CAD build for the part. Positions are in the model's coordinates, mm. Round coordinates to 2 decimals unless told otherwise and drop trailing zeros. Loops run counter-clockwise (first coordinate to the right, second up) from the corner with the lowest first, then second, coordinate; pieces in that order, holes last. Notation, with made-up numbers: (1.25, 47) - (9.25, 47) arc R28 ccw to (9.25, 67) - close; hole circle Ø10 at (50, 64). An arc over 180 degrees is marked (long way). Use one line per item in the form item = value.
from build123d import *

# Parameters (mm, degrees)
F0_R     = 1.5
F1_DEPTH = 1.5


with BuildPart() as f1:
    # F0 (on Top) → F1 (new body)
    with BuildSketch(Plane.XY):
        with BuildLine():
            ThreePointArc((-0.1201086231, 2.7473758241), (1.2696708079, 2.4393515613), (2.3192429637, 1.4777050029))
            Line((2.3192429637, 1.4777050029), (1.4660895902, 2.8167205482))
            Line((1.4660895902, 2.8167205482), (-0.1201086231, 2.7473758241))
        make_face()
        with BuildLine():
            Line((1.706306755, -2.6780311034), (2.4393515428, -1.2696708434))
            ThreePointArc((2.4393515428, -1.2696708434), (1.477704987, -2.3192429738), (0.1201085757, -2.7473758261))
            Line((0.1201085757, -2.7473758261), (1.706306755, -2.6780311034))
        make_face()
        with BuildLine():
            ThreePointArc((-2.4393515589, 1.2696708124), (-1.4777050217, 2.3192429516), (-0.1201086231, 2.7473758241))
            Line((-0.1201086231, 2.7473758241), (-1.706306755, 2.6780311034))
            Line((-1.706306755, 2.6780311034), (-2.4393515589, 1.2696708124))
        make_face()
        with BuildLine():
            ThreePointArc((2.3192429637, 1.4777050029), (2.6401153526, 0.7696043951), (2.75, 0))
            ThreePointArc((2.75, 0), (2.671209159, -0.6535607307), (2.4393515428, -1.2696708434))
            Line((2.4393515428, -1.2696708434), (3.1723963452, 0.1386894448))
            Line((3.1723963452, 0.1386894448), (2.3192429637, 1.4777050029))
        make_face()
        with BuildLine():
            Line((-1.4660895902, -2.8167205482), (0.1201085757, -2.7473758261))
            ThreePointArc((0.1201085757, -2.7473758261), (-1.2696708891, -2.439351519), (-2.3192430366, -1.4777048885))
            Line((-2.3192430366, -1.4777048885), (-1.4660895902, -2.8167205482))
        make_face()
        with BuildLine():
            ThreePointArc((-2.3192430366, -1.4777048885), (-2.7473758282, -0.1201085279), (-2.4393515589, 1.2696708124))
            Line((-2.4393515589, 1.2696708124), (-3.1723963452, -0.1386894448))
            Line((-3.1723963452, -0.1386894448), (-2.3192430366, -1.4777048885))
        make_face()
        with BuildLine():
            ThreePointArc((2.4393515428, -1.2696708434), (2.671209159, -0.6535607307), (2.75, 0))
            ThreePointArc((2.75, 0), (2.6401153526, 0.7696043951), (2.3192429637, 1.4777050029))
            ThreePointArc((2.3192429637, 1.4777050029), (1.2696708079, 2.4393515613), (-0.1201086231, 2.7473758241))
            ThreePointArc((-0.1201086231, 2.7473758241), (-1.4777050217, 2.3192429516), (-2.4393515589, 1.2696708124))
            ThreePointArc((-2.4393515589, 1.2696708124), (-2.7473758282, -0.1201085279), (-2.3192430366, -1.4777048885))
            ThreePointArc((-2.3192430366, -1.4777048885), (-1.2696708891, -2.439351519), (0.1201085757, -2.7473758261))
            ThreePointArc((0.1201085757, -2.7473758261), (1.477704987, -2.3192429738), (2.4393515428, -1.2696708434))
        make_face()
        Circle(F0_R, mode=Mode.SUBTRACT)
    extrude(amount=F1_DEPTH)


solid = f1.part
1) Slice it at B-B (y = 0.5). Write the cut outline in (x, z).
Report:
outline = (-2.84, 0) - (-1.41, 0) - (-1.41, 1.5) - (-2.84, 1.5) - close; (1.41, 0) - (2.94, 0) - (2.94, 1.5) - (1.41, 1.5) - close
2) Drill centre lines: probe 1 along X at (y, z) = (1.3, 0.1); probe 2 along X at (y, z) = (0.4, 0.45); probe 3 along Y at (x, z) = (0, 0.6). Where is each one in solid material? Low to high.
Report:
probe_1 = -2.42 to -0.75, 0.75 to 2.43
probe_2 = -2.89 to -1.45, 1.45 to 3.01
probe_3 = -2.75 to -1.5, 1.5 to 2.75
3) Slice it at D-D (x = 2). Write the cut outline in (y, z), plus the area to 3 significant figures.
Report:
outline = (-2.11, 0) - (1.98, 0) - (1.98, 1.5) - (-2.11, 1.5) - close
area = 6.14 mm^2
4) Slice it at C-C (x = 0.5). Write the cut outline in (y, z), plus the area to 3 significant figures.
Report:
outline = (-2.73, 0) - (-1.41, 0) - (-1.41, 1.5) - (-2.73, 1.5) - close; (1.41, 0) - (2.77, 0) - (2.77, 1.5) - (1.41, 1.5) - close
area = 4.02 mm^2
5) Two-plate mould, pull along Y, no slides. Class faces 1 (the cylindrical face through (-1.5, 0.07, 0.74)), 2 (the flat face through (-1.5, 0.7, 0)): +Y half, -Y half, draft (parallel to the pull), parting line (faces both ways), or undercut.
Report:
face_1 = undercut
face_2 = draft
6) Flat gauge pins, fed straight in: pin 1 (2.5 mm diameter, centred on x = 0, y = 0, fed in from +Z); pin 2 (1 mm diameter, centred on x = 0.5, y = 1, fed in from -Z). Where does each tip first touch, or does it go through?
Report:
pin_1 = through
pin_2 = 0
7) Slice it at A-A (z = 1.25). Write the cut outline in (x, y), plus the area to 3 significant figures.
Report:
outline = (-3.17, -0.14) - (-1.47, -2.82) - (1.71, -2.68) - (3.17, 0.14) - (1.47, 2.82) - (-1.71, 2.68) - close; hole circle Ø3 at (0, 0)
area = 19.1 mm^2
